Work out the finished part from the listing and answer in its coordinate system (mm). Face numbers are marked on the shaded views. A direction names the side the tool comes from. Round coordinates to 2 decimals unless told otherwise and drop trailing zeros. Order: outer loops, then holes, each group sorted by start corner. A loop starts at its lowest first (then second) coordinate and runs counter-clockwise, first axis right, second up. Notation, with made-up numbers: (18.25, -28.75) - (73.25, -28.75) arc R19 ccw to (73.25, -19.75) - close; hole circle Ø9 at (5.5, -32). An arc over 180 degrees is marked (long way). Put each result on its own line as item: value.
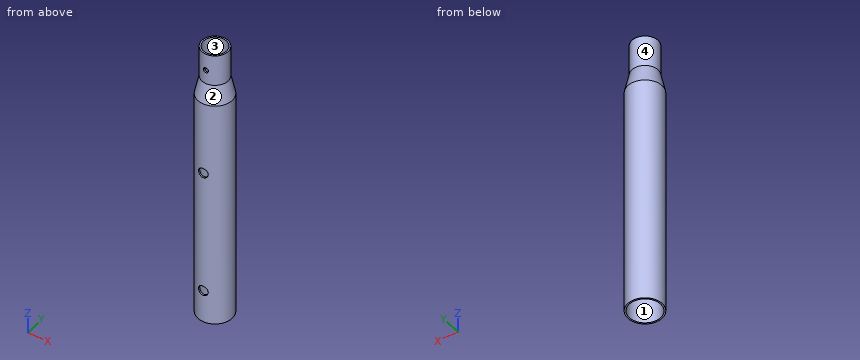
```python
from build123d import *

# Parameters (mm, degrees)
F0_R      = 13.2969
F1_DEPTH  = 31.75
F3_R      = 17.4625
F4_DEPTH  = 234.95
F4_FACE_R = 17.4625
F1_FACE_R = 13.2969
F6_T      = -1.524
F12_D     = 9.92124
F12_DEPTH = 6.35
F12_TIP   = 2.980641204
F13_D     = 5.159375
F13_DEPTH = 6.35
F13_TIP   = 1.5500326281


with BuildPart() as f1:
    # F0 (on Top) → F1 (new body)
    with BuildSketch(Plane.XY):
        Circle(F0_R)
    extrude(amount=-F1_DEPTH)



with BuildPart() as f4:
    # F3 (on offset) → F4 (new body)
    with BuildSketch(Plane.XY.offset(-285.75)):
        Circle(F3_R)
    extrude(amount=F4_DEPTH)


with BuildPart() as f1_1:
    add(f1.part)

    add(f4.part)  # F5 merges F4
    # F4_face (on face) → F5 section 0
    with BuildSketch(Plane.XY.offset(-50.8)):
        Circle(F4_FACE_R)
    # F1_face (on face) → F5 section 1
    with BuildSketch(Plane(origin=(0, 0, -31.75), x_dir=(1, 0, 0), z_dir=(0, 0, -1))):
        Circle(F1_FACE_R)
    loft()

    # F6
    f6_openings = [f1_1.faces().sort_by_distance(p)[0] for p in [
        (0, 0, 0),
        (0, 0, -285.75),
    ]]
    offset(amount=F6_T, openings=f6_openings, kind=Kind.INTERSECTION)

    # F12
    with Locations(Plane.XZ.offset(17.4625)):
        with Locations((0, -125.4125), (0, -252.4125)):
            Hole(F12_D / 2, depth=F12_DEPTH)
            with Locations((0, 0, -(F12_DEPTH + F12_TIP / 2))):  # 118° drill point
                Cone(0, F12_D / 2, F12_TIP, mode=Mode.SUBTRACT)

    # F13
    with Locations(Plane.XZ.offset(13.2969)):
        with Locations((0, -17.4625)):
            Hole(F13_D / 2, depth=F13_DEPTH)
            with Locations((0, 0, -(F13_DEPTH + F13_TIP / 2))):  # 118° drill point
                Cone(0, F13_D / 2, F13_TIP, mode=Mode.SUBTRACT)


solid = f1_1.part
```
1) Straight lines are drawn through the part: L1, parallel to Y at x = 0, z = -236; L2, parallel to X at y = -13.5, z = -227.5; L3, parallel to X at y = 2.5, z = -138. For each, find the intervals that lie inside material, in ascending order. Write a range as from..to.
Findings below:
L1: y = -17.46..-15.94, 15.94..17.46
L2: x = -11.08..-8.47, 8.47..11.08
L3: x = -17.28..-15.74, 15.74..17.28
2) For the marked faces 1 and 2, determine the directions among +Z, -Z, +X, -X, +Y, -Y from which every point of the face is accessible in a straight line to the end or side of a thin tool.
Findings below:
face 1: -Z
face 2: +Z
3) A cutting plane is placed at B-B on z = -141. Write down the section's boundary in (x, y) (1 decimal).
Findings below:
outline: circle Ø34.9 at (0, 0); hole circle Ø31.9 at (0, 0)
4) A cutting plane is placed at A-A on x = 0. Write down the section's boundary in (y, z), then the cut area to 3 significant figures.
Findings below:
outline: (-17.46, -285.75) - (-15.94, -285.75) - (-15.94, -257.37) - (-17.46, -257.37) - close; (-17.46, -247.45) - (-15.94, -247.45) - (-15.94, -130.37) - (-17.46, -130.37) - close; (-17.46, -120.45) - (-15.94, -120.45) - (-15.94, -50.96) - (-11.77, -31.91) - (-11.77, -20.04) - (-13.3, -20.04) - (-13.3, -31.75) - (-17.46, -50.8) - close; (-13.3, -14.88) - (-11.77, -14.88) - (-11.77, 0) - (-13.3, 0) - close; (11.77, -31.91) - (15.94, -50.96) - (15.94, -285.75) - (17.46, -285.75) - (17.46, -50.8) - (13.3, -31.75) - (13.3, 0) - (11.77, 0) - close
area: 834 mm2
5) Given pin 1 Ø6.5 at (x, z) = (0, -17.46) entering from +Y; pin 2 Ø1 at (y, z) = (6, -186) entering from +X; pin 3 Ø1 at (y, z) = (13.5, -127.5) entering from +X, each flat-ended and moving along its own axis, determine where each tip first touches the part or whether it passes through.
Findings below:
pin 1: stops at y = 13.3
pin 2: stops at x = 16.57
pin 3: stops at x = 11.66
6) For a pull along X with two mould halves and no side action, classify the marked faces 3 and 4 as pulls with the +X half, pulls with the -X half, needs draft (parallel to the pull), parting line crosses it, or undercut.
Findings below:
face 3: undercut
face 4: parting line crosses it
